Geometry check sheet. Reference: drawing and pictorial views, mm from the part's lowest x, y, z. A direction names the side the tool comes from. Coordinates: 2 decimals unless noted, no trailing zeros. Loops run counter-clockwise (first coordinate to the right, second up) from the corner with the lowest first, then second, coordinate; pieces in that order, holes last. Notation, with made-up numbers: (2, 4) -> (55, 4) arc R31 cw to (55, 35) -> close; hole circle Ø9 at (-16.5, -29.5). An arc over 180 degrees is marked (long way). Answer as a JSON object with one key per item and string values. Group by question number.
Q1. Cross-section at A-A on y = 19.05. Record the boundary of the cut face in (x, z), and give its area (3 significant figures).
Q2. Cross-section at D-D on x = 26.5. Record the boundary of the cut face in (y, z).
Q3. Gauge pin test, flat ends, axial feed: pin 1 Ø3 at (y, z) = (12.5, 9.5) entering from -X; pin 2 Ø4 at (x, y) = (19.5, 32.5) entering from -Z; pin 3 Ø4 at (x, z) = (10, 2) entering from -Y; pin 4 Ø4 at (x, z) = (21.5, 7.5) entering from +Y (3 decimals). Record the tip position at first contact, or that the pin passes through.
Q4. Scan lines: L1, parallel to Z at x = 36, y = 14; L2, parallel to Y at x = 19.05, z = 11.25; L3, parallel to Y at x = 24, z = 4 (1 decimal). Record each from-to range of solid material in increasing order.
Q5. Set-up check for the marked faces 4 and 5: record each of +Z, -Z, +X, -X, +Y, -Y from which the full face is reachable in a straight line by a thin tool's end or side.
Q6. Cross-section at C-C on z = 5.25. Record the boundary of the cut face in (x, y), and give its area (3 significant figures).
Q7. Release check for a two-part mould opening along Z. For the marked faces 1, 2 and 3 record: released by +Z, released by -Z, zero draft, split by the parting line, or undercut.
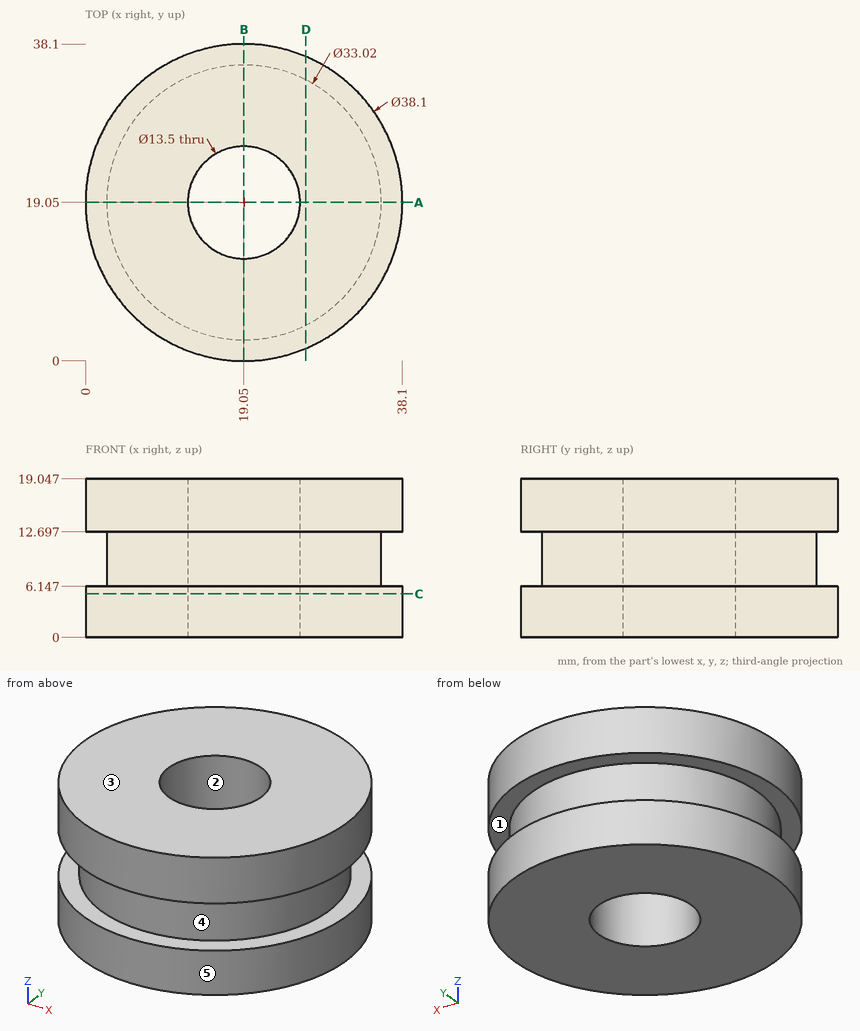
Computed values:
{
 "1": {"outline": "(0, 0) -> (12.3, 0) -> (12.3, 19.05) -> (0, 19.05) -> (0, 12.7) -> (2.54, 12.7) -> (2.54, 6.15) -> (0, 6.15) -> close; (25.8, 0) -> (38.1, 0) -> (38.1, 6.15) -> (35.56, 6.15) -> (35.56, 12.7) -> (38.1, 12.7) -> (38.1, 19.05) -> (25.8, 19.05) -> close", "area": "435 mm²"},
 "2": {"outline": "(1.52, 0) -> (36.58, 0) -> (36.58, 6.15) -> (33.78, 6.15) -> (33.78, 12.7) -> (36.58, 12.7) -> (36.58, 19.05) -> (1.52, 19.05) -> (1.52, 12.7) -> (4.32, 12.7) -> (4.32, 6.15) -> (1.52, 6.15) -> close"},
 "3": {"pin 1": "stops at x = 3.33", "pin 2": "stops at z = 0", "pin 3": "stops at y = 1.35", "pin 4": "stops at y = 38.075"},
 "4": {"L1": "z = 0 to 6.15, 12.7 to 19.05", "L2": "y = 2.54 to 12.3, 25.8 to 35.56", "L3": "y = 0.7 to 14.5, 23.6 to 37.4"},
 "5": {"face 4": "none", "face 5": "+Z, -Z"},
 "6": {"outline": "circle Ø38.1 at (19.05, 19.05); hole circle Ø13.5 at (19.05, 19.05)", "area": "997 mm²"},
 "7": {"face 1": "undercut", "face 2": "zero draft", "face 3": "released by +Z"}
}
